The listing builds one solid part. Answer for the finished solid, in the listing's coordinates (mm). Face numbers are marked on the shaded views. A direction names the side the tool comes from. Coordinates: 2 decimals unless noted, no trailing zeros. Order: outer loops, then holes, each group sorted by start corner. A loop starts at its lowest first (then second) coordinate and runs counter-clockwise, first axis right, second up. Notation, with made-up numbers: (-37, -17.5) -> (-12, -17.5) arc R8 ccw to (-12, -5.5) -> close; hole circle Ø1 at (23.25, 62.25). An arc over 180 degrees is marked (long way). Answer in a Markdown table with one row per item.
```python
from build123d import *

# Parameters (mm, degrees)
SKETCH1_R           = 2.8
BOSS_EXTRUDE1_DEPTH = 0.6
SKETCH2_W           = 1.5
SKETCH2_H           = 1.5
BOSS_EXTRUDE2_DEPTH = 8
SKETCH6_R           = 2.25
BOSS_EXTRUDE3_DEPTH = 7
CUT_EXTRUDE1_DEPTH  = 103.8
SKETCH9_R           = 1.75
CUT_EXTRUDE3_DEPTH  = 10


with BuildPart() as part:
    # Sketch1 → Boss-Extrude1 (new body)
    with BuildSketch(Plane(origin=(0, 0, 0), x_dir=(1, 0, 0), z_dir=(0, 1, 0))):
        Circle(SKETCH1_R)
    extrude(amount=BOSS_EXTRUDE1_DEPTH)

    # Sketch2 → Boss-Extrude2 (add)
    with BuildSketch(Plane(origin=(0, 0.6, 0), x_dir=(1, 0, 0), z_dir=(0, 1, 0))):
        with BuildLine():
            Line((0.75, 0.75), (0.75, -0.75))
            Line((0.75, -0.75), (2, -0.75))
            ThreePointArc((2, -0.75), (2.75, 0), (2, 0.75))
            Line((2, 0.75), (0.75, 0.75))
        make_face()
        with BuildLine():
            Line((-0.75, 2), (-0.75, 0.75))
            Line((-0.75, 0.75), (0.75, 0.75))
            Line((0.75, 0.75), (0.75, 2))
            ThreePointArc((0.75, 2), (0, 2.75), (-0.75, 2))
        make_face()
        Rectangle(SKETCH2_W, SKETCH2_H)
        with BuildLine():
            Line((-2, -0.75), (-0.75, -0.75))
            Line((-0.75, -0.75), (-0.75, 0.75))
            Line((-0.75, 0.75), (-2, 0.75))
            ThreePointArc((-2, 0.75), (-2.75, 0), (-2, -0.75))
        make_face()
        with BuildLine():
            Line((-0.75, -0.75), (-0.75, -2))
            ThreePointArc((-0.75, -2), (0, -2.75), (0.75, -2))
            Line((0.75, -2), (0.75, -0.75))
            Line((0.75, -0.75), (-0.75, -0.75))
        make_face()
    extrude(amount=BOSS_EXTRUDE2_DEPTH)

    # Sketch6 → Boss-Extrude3 (add)
    with BuildSketch(Plane.XZ):
        Circle(SKETCH6_R)
    extrude(amount=BOSS_EXTRUDE3_DEPTH)

    # Sketch7 → Cut-Extrude1 (cut, through all)
    with BuildSketch(Plane.XY.offset(100)):
        with BuildLine():
            Line((0.5, -5), (0.5, -6.962153423))
            ThreePointArc((0.5, -6.962153423), (0, -7.462153423), (-0.5, -6.962153423))
            Line((-0.5, -6.962153423), (-0.5, -5))
            ThreePointArc((-0.5, -5), (0, -4.5), (0.5, -5))
        make_face()
    extrude(amount=-CUT_EXTRUDE1_DEPTH, mode=Mode.SUBTRACT)

    # Sketch9 → Cut-Extrude3 (cut)
    with BuildSketch(Plane(origin=(0, -10, 0), x_dir=(1, 0, 0), z_dir=(0, 1, 0))):
        Circle(SKETCH9_R)
    extrude(amount=CUT_EXTRUDE3_DEPTH, mode=Mode.SUBTRACT)


solid = part.part
```
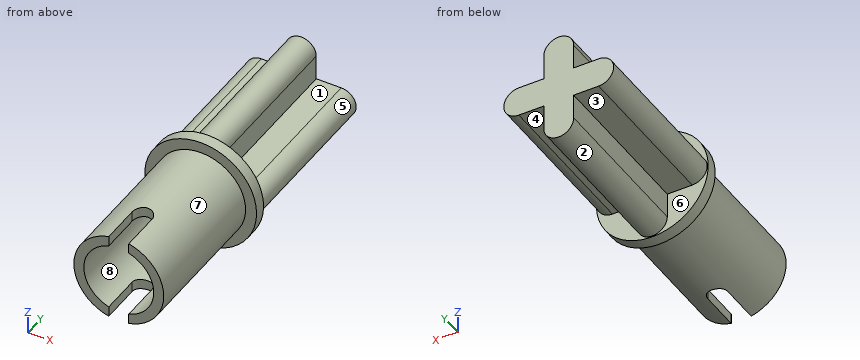
(1) A cutting plane is placed at D-D, the plane y = -1. Determine the outline of the cut face in (x, z), then the cut area to 3 significant figures.
Check values:
| item | result |
|---|---|
| outline | circle Ø4.5 at (0, 0); hole circle Ø3.5 at (0, 0) |
| area | 6.28 mm² |
(2) A cutting plane is placed at C-C, the plane y = 5. Determine the outline of the cut face in (x, z), then the cut area to 3 significant figures.
Check values:
| item | result |
|---|---|
| outline | (-2, -0.75) -> (-0.75, -0.75) -> (-0.75, -2) arc R0.75 ccw to (0.75, -2) -> (0.75, -0.75) -> (2, -0.75) arc R0.75 ccw to (2, 0.75) -> (0.75, 0.75) -> (0.75, 2) arc R0.75 ccw to (-0.75, 2) -> (-0.75, 0.75) -> (-2, 0.75) arc R0.75 ccw to start |
| area | 13.3 mm² |
(3) A cutting plane is placed at A-A, the plane z = 0. Determine the outline of the cut face in (x, y), then the cut area to 3 significant figures.
Check values:
| item | result |
|---|---|
| outline | (-2.8, 0) -> (-2.25, 0) -> (-2.25, -7) -> (-1.75, -7) -> (-1.75, 0) -> (1.75, 0) -> (1.75, -7) -> (2.25, -7) -> (2.25, 0) -> (2.8, 0) -> (2.8, 0.6) -> (2.75, 0.6) -> (2.75, 8.6) -> (-2.75, 8.6) -> (-2.75, 0.6) -> (-2.8, 0.6) -> close |
| area | 54.4 mm² |
(4) Find the intervals of material crossed by line 1 along X through (y, z) = (-3.75, 0); line 2 along Y through (x, z) = (-1.1, -0.45), in increasing order. Write a range as from..to.
Check values:
| item | result |
|---|---|
| line 1 | -2.25..-1.75, 1.75..2.25 |
| line 2 | 0..8.6 |
(5) A cutting plane is placed at B-B, the plane x = 0. Determine the outline of the cut face in (y, z), then the cut area to 3 significant figures.
Check values:
| item | result |
|---|---|
| outline | (-4.5, -2.25) -> (0, -2.25) -> (0, -2.8) -> (0.6, -2.8) -> (0.6, -2.75) -> (8.6, -2.75) -> (8.6, 2.75) -> (0.6, 2.75) -> (0.6, 2.8) -> (0, 2.8) -> (0, 2.25) -> (-4.5, 2.25) -> (-4.5, 1.75) -> (0, 1.75) -> (0, -1.75) -> (-4.5, -1.75) -> close |
| area | 51.9 mm² |
(6) Which of the six approach directions +Z, -Z, +X, -X, +Y, -Y give full straight-line access (tool end or side, diameter ignored) to the marked faces 1, 2, 3, 4 and 5?
Check values:
| item | result |
|---|---|
| face 1 | +Z, +X, +Y |
| face 2 | -Z, +Y |
| face 3 | -Z, -X, +Y |
| face 4 | -Z, +X, +Y |
| face 5 | +X, +Y |
(7) Flat-ended cylindrical pins translate along their axes: pin 1 (0.6 mm diameter, centred on x = -1.5, y = 5.5, fed in from +Z); pin 2 (1 mm diameter, centred on y = 3, z = -1.5, fed in from -X); pin 3 (1.5 mm diameter, centred on x = 1, y = 3.5, fed in from -Z). Find the tip coordinate at first contact, or state that the pin passes through.
Check values:
| item | result |
|---|---|
| pin 1 | z = 0.75 |
| pin 2 | x = -0.75 |
| pin 3 | z = -2.71 |
(8) For a pull along X with two mould halves and no side action, classify the marked faces 6, 7 and 8 as released by +X, released by -X, zero draft, split by the parting line, or undercut.
Check values:
| item | result |
|---|---|
| face 6 | zero draft |
| face 7 | split by the parting line |
| face 8 | undercut |
